Here's how the part is built. I have some questions about the finished solid (model axes, mm). Coordinates: 2 decimals unless noted, no trailing zeros. Loops run counter-clockwise (first coordinate to the right, second up) from the corner with the lowest first, then second, coordinate; pieces in that order, holes last. Notation, with made-up numbers: (80.5, -3.75) - (126.5, -3.75) arc R8 ccw to (126.5, 7.25) - close; hole circle Ø7 at (27, -11.5). An arc over 180 degrees is marked (long way). Use a Markdown table: item, result.
```python
from build123d import *

# Parameters (mm, degrees)
CROQUIS1_R              = 3.75
CROQUIS1_R_2            = 2
CROQUIS1_R_3            = 2.5
SALIENTE_EXTRUIR1_DEPTH = 6.35
CROQUIS2_R              = 7
CROQUIS2_R_2            = 2.5
CORTAR_EXTRUIR1_DEPTH   = 10


with BuildPart() as part:
    # Croquis1 → Saliente-Extruir1 (new body)
    with BuildSketch(Plane.XY):
        with BuildLine():
            Line((0, 0), (-110, 0))
            Line((-110, 0), (-110, 124))
            Line((-110, 124), (-95.487652439, 124))
            ThreePointArc((-95.487652439, 124), (-55, 84.5), (-14.512347561, 124))
            Line((-14.512347561, 124), (0, 124))
            Line((0, 124), (0, 0))
        make_face()
        with Locations((-93, 97)):
            Circle(CROQUIS1_R, mode=Mode.SUBTRACT)
        with Locations((-84.75, 67)):
            Circle(CROQUIS1_R_2, mode=Mode.SUBTRACT)
        with Locations((-25.25, 67)):
            Circle(CROQUIS1_R_2, mode=Mode.SUBTRACT)
        with Locations((-17, 97)):
            Circle(CROQUIS1_R, mode=Mode.SUBTRACT)
        with Locations((-99.75, 14.601014199)):
            Circle(CROQUIS1_R_3, mode=Mode.SUBTRACT)
        with Locations((-10.25, 14.601014199)):
            Circle(CROQUIS1_R_3, mode=Mode.SUBTRACT)
    extrude(amount=SALIENTE_EXTRUIR1_DEPTH)

    # Croquis2 → Cortar-Extruir1 (cut)
    with BuildSketch(Plane.XY.offset(6.35)):
        with Locations((-55, 26.601014199)):
            Circle(CROQUIS2_R)
        with Locations((-40, 11.601014199)):
            Circle(CROQUIS2_R_2)
        with Locations((-70, 11.601014199)):
            Circle(CROQUIS2_R_2)
        with Locations((-70, 41.601014199)):
            Circle(CROQUIS2_R_2)
        with Locations((-40, 41.601014199)):
            Circle(CROQUIS2_R_2)
    extrude(amount=-CORTAR_EXTRUIR1_DEPTH, mode=Mode.SUBTRACT)


solid = part.part
```
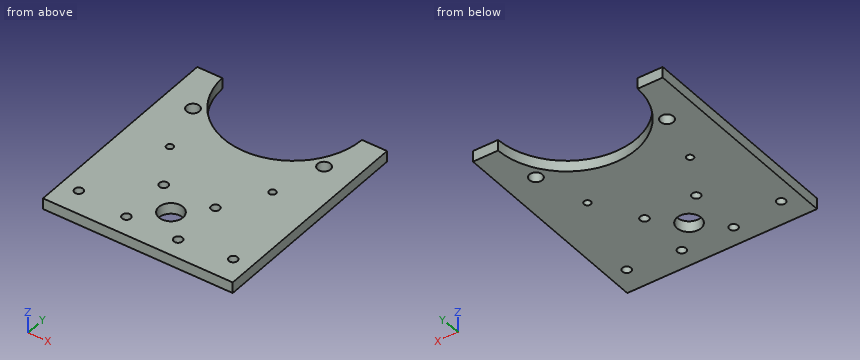
Q1. Will these pins go through, and if not, where does the flat tip stop? P1, Ø3.5, axis at x = -84.75, y = 67, coming from the -Z side; P2, Ø1, axis at x = -49, z = 4, coming from the +Y side (3 decimals).
Check values:
| item | result |
|---|---|
| P1 | through |
| P2 | y = 85.025 |
Q2. Please list where these lines run through material, in increasing order: L1, parallel to X at y = 14.5, z = 2.75; L2, parallel to Y at x = -10.25, z = 3; L3, parallel to Y at x = -55, z = 4. Write a range as from..to.
Check values:
| item | result |
|---|---|
| L1 | -110..-102.25, -97.25..-12.75, -7.75..0 |
| L2 | 0..12.1, 17.1..124 |
| L3 | 0..19.6, 33.6..84.5 |
Q3. I want a section at B-B, the plane y = 97. Write out the boundary of the cut face in (x, z), then the cut area to 3 significant figures.
Check values:
| item | result |
|---|---|
| outline | (-110, 0) - (-96.75, 0) - (-96.75, 6.35) - (-110, 6.35) - close; (-89.25, 0) - (-84.26, 0) - (-84.26, 6.35) - (-89.25, 6.35) - close; (-25.74, 0) - (-20.75, 0) - (-20.75, 6.35) - (-25.74, 6.35) - close; (-13.25, 0) - (0, 0) - (0, 6.35) - (-13.25, 6.35) - close |
| area | 232 mm^2 |
Q4. I want a section at A-A, the plane x = -99.75. Write out the boundary of the cut face in (y, z), then the cut area to 3 significant figures.
Check values:
| item | result |
|---|---|
| outline | (0, 0) - (12.1, 0) - (12.1, 6.35) - (0, 6.35) - close; (17.1, 0) - (124, 0) - (124, 6.35) - (17.1, 6.35) - close |
| area | 756 mm^2 |
Q5. I want a section at D-D, the plane x = -55. Write out the boundary of the cut face in (y, z).
Check values:
| item | result |
|---|---|
| outline | (0, 0) - (19.6, 0) - (19.6, 6.35) - (0, 6.35) - close; (33.6, 0) - (84.5, 0) - (84.5, 6.35) - (33.6, 6.35) - close |
Q6. I want a section at C-C, the plane z = 4.25. Give the number of separate pieces and of enclosed holes in the cut face, then the cut area to 3 significant figures.
Check values:
| item | result |
|---|---|
| separate pieces | 1 |
| enclosed holes | 11 |
| area | 10,800 mm^2 |
